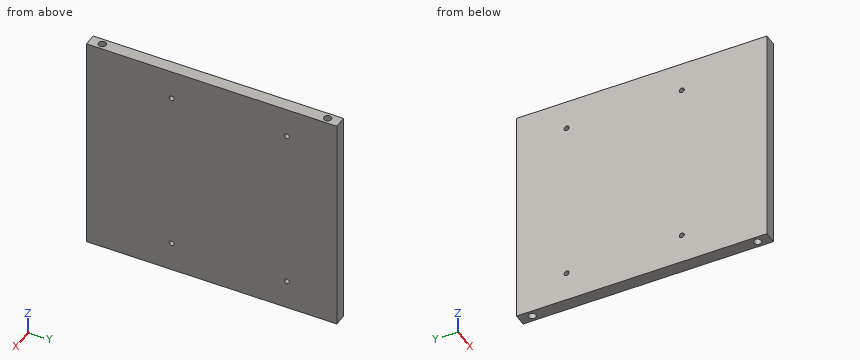
Autodesk Inventor part; units mm, degrees
ref_plane "YZ Plane" through (0, 0, 0) normal (1, 0, 0) x (0, 1, 0)
ref_plane "XZ Plane" through (0, 0, 0) normal (0, 1, 0) x (-1, 0, 0)
ref_plane "XY Plane" through (0, 0, 0) normal (0, 0, 1) x (1, 0, 0)
sketch "Boceto1" plane through (0, 0, 0) normal (1, 0, 0) x (0, 1, 0)
  line L0 (0, 0) -> (-100, 0)
  line L1 (-100, 0) -> (-100, -90)
  line L2 (-100, -90) -> (0, -90)
  line L3 (0, -90) -> (0, 0)
  dimension "d0" = 90
  dimension "d1" = 100
extrude "Extrusión1" add sketch "Boceto1" along normal blind 5
sketch "Boceto2" plane through (0, -100, 0) normal (0, 0, 1) x (1, 0, 0)
  line L0 (20, -20) -> (0, 0)
  line L1 (20, -20) -> (20, -15)
  line L2 (20, -15) -> (5, 0)
  line L3 (0, 0) -> (0, 100)
  line L4 (0, 0) -> (5, 0)
  dimension "d6" = 5
extrude "Extrusión2" add sketch "Boceto2" against normal blind 90
sketch "Boceto3" plane through (5, 0, -90) normal (0, 0, -1) x (-1, 0, 0)
  circle A0 centre (2.5, -5) radius 1.5
  circle A1 centre (2.5, -95) radius 1.5
  line L0 (5, -100) -> (5, 0)
  line L1 (5, 0) -> (0, 0)
  line L2 (0, -100) -> (0, 0)
  dimension "d9" = 3
  dimension "d10" = 3
  dimension "d11" = 2.5
  dimension "d12" = 5
  dimension "d13" = 5
  dimension "d14" = 2.5
extrude "Extrusión3" cut sketch "Boceto3" against normal blind 3
sketch "Boceto4" plane through (0, 0, 0) normal (0, 0, 1) x (1, 0, 0)
  circle A0 centre (2.5, -5) radius 1.5
  circle A1 centre (2.5, -5) radius 1.5
  circle A2 centre (2.5, -95) radius 1.5
  circle A3 centre (2.5, -95) radius 1.5
  point P0 (0, 0)
extrude "Extrusión4" cut sketch "Boceto4" against normal blind 3
sketch "Boceto5" plane through (0, 0, 0) normal (0, 0, 1) x (1, 0, 0)
  line L0 (0, 0) -> (0, -100)
  line L1 (20, -115) -> (5, -100)
  line L2 (0, -100) -> (5, -100)
  line L3 (5, -100) -> (2.5, -102.5)
  line L4 (0, -100) -> (20, -120)
extrude "Extrusión5" cut sketch "Boceto5" against normal blind 3000
sketch "Boceto6" plane through (5, 0, 0) normal (1, 0, 0) x (0, 0, -1)
  point P0 (0, 0)
sketch "Boceto7" plane through (20, -120, 0) normal (0, 0, 1) x (1, 0, 0)
  line L0 (-17.5, 17.5) -> (0, 0)
  line L1 (0, 5) -> (-15, 20)
  line L2 (-17.5, 17.5) -> (-15, 20)
  line L3 (0, 0) -> (0, 5)
  line L4 (-15, 20) -> (0, 5)
  line L5 (0, 5) -> (0, 0)
  line L6 (0, 0) -> (-17.5, 17.5)
  point P0 (-20, 120)
extrude "Extrusión6" cut sketch "Boceto7" against normal blind 3000
sketch "Boceto8" plane through (5, 0, 0) normal (1, 0, 0) x (0, 0, -1)
  circle A0 centre (12, -20) radius 1
  line L0 (0, 0) -> (0, -100)
  line L1 (90, 0) -> (0, 0)
  circle A1 centre (78, -20) radius 1
  circle A2 centre (12, -66) radius 1
  circle A3 centre (78, -66) radius 1
  dimension "d23" = 2
  dimension "d24" = 12
  dimension "d25" = 20
  dimension "d26" = 2
  dimension "d27" = 66
  dimension "d28" = 20
  dimension "d29" = 2
  dimension "d30" = 2
  dimension "d31" = 46
  dimension "d32" = 46
  dimension "d33" = 66
extrude "Extrusión7" cut sketch "Boceto8" against normal blind 5
properties part number "Atras"
The listing builds one solid part. Answer for the finished solid, in the listing's coordinates (mm). Give positions to 0.01 mm unless a question says otherwise; leave off trailing zeros. Order: outer loops, then holes, each group sorted by start corner. A loop starts at its lowest first (then second) coordinate and runs counter-clockwise, first axis right, second up. Notation, with made-up numbers: (32.5, 53) -> (59.5, 53) arc R15 cw to (59.5, 76) -> close; hole circle Ø11 at (57.25, -11.75). An arc over 180 degrees is marked (long way). Put each result on its own line as item: value.
Item 1: A cutting plane is placed at A-A on y = -95. Give the vertices of the cut face in (x, z).
Established:
outline: (0, -90) -> (1, -90) -> (1, -87) -> (4, -87) -> (4, -90) -> (5, -90) -> (5, 0) -> (4, 0) -> (4, -3) -> (1, -3) -> (1, 0) -> (0, 0) -> close
Item 2: Straight lines are drawn through the part: line 1 (Y direction, x = 2.5, z = -88.6); line 2 (Y direction, x = 2.4, z = -78); line 3 (Z direction, x = 1.55, y = -66). For each, find the intervals that lie inside material, in ascending order.
Established:
line 1: y = -100 to -96.5, -93.5 to -6.5, -3.5 to 0
line 2: y = -100 to -67, -65 to -21, -19 to 0
line 3: z = -90 to -79, -77 to -13, -11 to 0
Item 3: Given P1, Ø2.5, axis at y = -20, z = -78, coming from the +X side; P2, Ø1.5, axis at x = 2, y = -5.5, coming from the -Z side; P3, Ø1.5, axis at x = 2.5, y = -94.5, coming from the +Z side; P4, Ø1.2, axis at y = -66, z = -12, coming from the -X side, each flat-ended and moving along its own axis, determine where each tip first touches the part or whether it passes through.
Established:
P1: stops at x = 5
P2: stops at z = -87
P3: stops at z = -3
P4: passes through
